from build123d import *

# Parameters (mm, degrees)
F0_W     = 888.9909996986
F0_H     = 5.1128612518
F1_DEPTH = 25.4
F3_DEPTH = 12.7
F5_DEPTH = 25.4


with BuildPart() as f1:
    # F0 (on Top) → F1 (new body)
    with BuildSketch(Plane.XY):
        Polygon((444.5, -109.1871387482), (444.5, 114.3), (-444.5, 114.3), (-444.5, -114.3), (-444.4909996986, -114.3), (-444.4909996986, -109.1871387482), align=None)
        Polygon((444.5090003014, -109.1871387482), (444.5, -109.1871387482), (444.5, -114.3), (-444.4909996986, -114.3), (-444.4909996986, -337.7871387482), (444.5090003014, -337.7871387482), align=None)
        with Locations((0.0045001507, -111.7435693741)):
            Rectangle(F0_W, F0_H)
    extrude(amount=F1_DEPTH)

    # F2 (on face) → F3 (cut)
    with BuildSketch(Plane.XY.offset(25.4)):
        Polygon((-266.7, 114.3), (-279.4, 114.3), (-279.4, -337.7871387482), (-254, -337.7871387482), (-254, 114.3), align=None)
    extrude(amount=-F3_DEPTH, mode=Mode.SUBTRACT)

    # F4 (on face) → F5 (cut)
    with BuildSketch(Plane(origin=(0, 0, 0), x_dir=(1, 0, 0), z_dir=(0, 0, -1))):
        with BuildLine():
            Line((-444.5, 114.3), (-444.5, -91.3470163941))
            add(Edge.make_bspline(
                [(-444.5, -91.3470163941), (-439.8643107844, -70.3071791015), (-396.5612558672, 10.0595120676), (-272.6729040405, 121.5892977787), (-374.2433991601, 303.6629585996), (-343.9956112011, 329.4717163372), (-334.2497050762, 337.7871387482)],
                knots=[0.1020972669, 0.1020972669, 0.1020972669, 0.1020972669, 0.3199118394, 0.5865273881, 0.8667797776, 1, 1, 1, 1], degree=3))
            Line((-334.2497050762, 337.7871387482), (-444.4909996986, 337.7871387482))
            Line((-444.4909996986, 337.7871387482), (-444.4909996986, 114.3))
            Line((-444.4909996986, 114.3), (-444.5, 114.3))
        make_face()
    extrude(amount=-F5_DEPTH, mode=Mode.SUBTRACT)


solid = f1.part
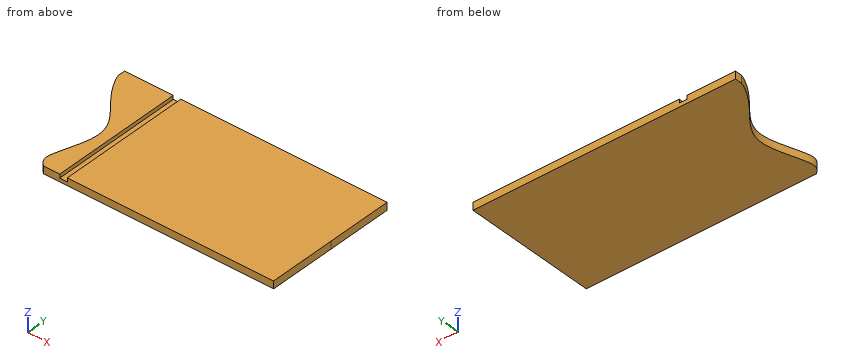
Read the model definition and answer for the solid it produces. Units are mm, in the model's axes. Give positions to 0.01 mm unless a question says otherwise; leave off trailing zeros. Write each loop counter-clockwise with the first axis right and the second up, starting at its lowest first coordinate (ties: lowest second). Pieces come first, ordered by that corner, then holes. Notation, with made-up numbers: (45.25, 2.5) - (69.25, 2.5) arc R20 cw to (69.25, 24.5) - close; hole circle Ø8 at (80, 38). An arc over 180 degrees is marked (long way). Use CSV: the item, a comma, the result in double quotes. Start each with the question number.
(1) Consider line 1 along X through (y, z) = (-267.5, 20.25); line 2 along X through (y, z) = (-15.5, 14.5); line 3 along Y through (x, z) = (-405, 23.25). Determine where each line is inside the solid, lowest interval first.
(2) Given P1, Ø4, axis at y = -25.5, z = 21.5, coming from the -X side; P2, Ø1, axis at x = -211, y = -39, coming from the -Z side; P3, Ø12.5, axis at y = 39, z = 17.5, coming from the +X side; P4, Ø1.5, axis at y = -127.5, z = 22, coming from the -X side, each flat-ended and moving along its own axis, determine where each tip first touches the part or whether it passes through.
(3) Find section A-A (x = -263). Give the vertices of the cut face in (y, z), plus the area to 3 significant figures.
Findings below:
1,line 1,"-346.76 to -279.4, -254 to 444.51"
1,line 2,"-381.28 to -279.4, -254 to 444.5"
1,line 3,"15.07 to 114.3"
2,P1,"x = -374.59"
2,P2,"z = 0"
2,P3,"x = 444.5"
2,P4,"x = -316.14"
3,outline,"(-337.79, 0) - (114.3, 0) - (114.3, 12.7) - (-337.79, 12.7) - close"
3,area,"5,740 mm2"
